Autodesk Inventor part; units mm, degrees
ref_plane "YZ Plane" through (0, 0, 0) normal (1, 0, 0) x (0, 1, 0)
ref_plane "XZ Plane" through (0, 0, 0) normal (0, 1, 0) x (-1, 0, 0)
ref_plane "XY Plane" through (0, 0, 0) normal (0, 0, 1) x (1, 0, 0)
sketch "Sketch1" plane through (0, 0, 0) normal (0, 1, 0) x (-1, 0, 0)
  line L0 (0, 0) -> (-359.4604, 0)
  line L1 (-173.205, -100) -> (23.0868, -100)
  line L2 (23.0868, -100) -> (-382.5472, -100)
  line L3 (-382.5472, -100) -> (-359.4604, 0)
  line L4 (23.0868, -100) -> (0, 0)
  dimension "d16" = 103
  dimension "d17" = 100
  dimension "d18" = 405.634
  dimension "d19" = 103
extrude "Extrusion1" add sketch "Sketch1" along normal blind 5
sketch "Sketch2" plane through (0, 5, 0) normal (0, 1, 0) x (1, 0, 0)
  line L0 (-23.0868, 100) -> (0, 0)
  line L1 (0, 0) -> (-23.0868, 100)
  line L2 (382.5472, 100) -> (-23.0868, 100)
  line L3 (-23.0868, 100) -> (382.5472, 100)
  line L4 (359.4604, 0) -> (382.5472, 100)
  line L5 (382.5472, 100) -> (359.4604, 0)
  line L6 (359.4604, 0) -> (0, 0)
  line L7 (3.9772, 5) -> (-16.801, 95)
  line L8 (-16.801, 95) -> (376.2613, 95)
  line L9 (376.2613, 95) -> (355.4832, 5)
  line L10 (355.4832, 5) -> (3.9772, 5)
  dimension "d6" = 5
extrude "Extrusion2" add sketch "Sketch2" along normal blind 90
sketch "Sketch3" plane through (0, 0, 0) normal (0, 0, 1) x (1, 0, 0)
  line L0 (0, 0) -> (0, 50)
  line L1 (0, 0) -> (0, 95)
  line L2 (0, 50) -> (345.363, 50)
  circle A0 centre (172.6815, 50) radius 7.5
  dimension "d9" = 50
  dimension "d10" = 15
extrude "Extrusion3" cut sketch "Sketch3" against normal blind 455
sketch "Sketch4" plane through (0, 95, 0) normal (0, 1, 0) x (1, 0, 0)
  line L0 (-23.0868, 100) -> (0, 0)
  line L1 (0, 0) -> (-23.0868, 100)
  line L2 (359.4604, 0) -> (382.5472, 100)
  line L3 (-23.0868, 100) -> (382.5472, 100)
  line L4 (382.5472, 100) -> (359.4604, 0)
  line L5 (359.4604, 0) -> (0, 0)
  line L6 (355.4832, 5) -> (3.9772, 5)
extrude "Extrusion4" add sketch "Sketch4" along normal blind 5
properties part number "v chasis" material "Steel, Mild"
Can you work these out from the model? Positions are in its coordinate system, mm. A direction names the side the tool comes from. Give positions to 0.01 mm unless a question says otherwise; leave off trailing zeros. Write each loop counter-clockwise with the first axis right and the second up, starting at its lowest first coordinate (ties: lowest second). Pieces come first, ordered by that corner, then holes. Notation, with made-up numbers: (-8.75, 51) -> (11.25, 51) arc R19 cw to (11.25, 75) -> close; hole circle Ø1 at (-21.75, 80). An arc over 180 degrees is marked (long way). One line per item, written item: value.
Q1. We'd pull the mould along X, two halves only. Please class faces 1 (the face through (370.842, 49.3, -49.3)), 2 (the face through (183, 0, -49)), 3 (the face through (366.018, 49.37, -50.63)): +X half, -X half, draft (parallel to the pull), parting line (faces both ways), or undercut.
Results found:
face 1: +X half
face 2: draft
face 3: undercut
Q2. Imagine slicing it at A-A on y = 50. Please give me the cut outline in (x, z).
Results found:
outline: (-23.09, -100) -> (165.18, -100) -> (165.18, -95) -> (-16.8, -95) -> (3.98, -5) -> (165.18, -5) -> (165.18, 0) -> (0, 0) -> close; (180.18, -100) -> (382.55, -100) -> (359.46, 0) -> (180.18, 0) -> (180.18, -5) -> (355.48, -5) -> (376.26, -95) -> (180.18, -95) -> close
Q3. For P1, Ø1.5, axis at y = 58.5, z = -40, coming from the +X side; P2, Ø4, axis at y = 22, z = -77, coming from the -X side; P3, Ø4, axis at y = 64.5, z = -38, coming from the +X side, each with a flat end and sliding along its axis, tell me the tip position at first contact or that it passes through.
Results found:
P1: stops at x = 368.87
P2: stops at x = -18.24
P3: stops at x = 368.7
Q4. Which directions (+Z, -Z, +X, -X, +Y, -Y) give clear straight access to the entire face, cutting with the end or side of a thin tool? Please do faces 4 (the face through (-6.266, 49.37, -49.37)), 5 (the face through (177, 38, -100)).
Results found:
face 4: none
face 5: -Z, +X, -X, +Y, -Y
Q5. Please list where these lines run through material, in increasing order: line 1 (Z direction, x = 326.5, y = 81); line 2 (Y direction, x = 304.5, z = -15); line 3 (X direction, y = 50, z = -2.75). Write a range as [from, to].
Results found:
line 1: z = [-100, -95], [-5, 0]
line 2: y = [0, 5], [95, 100]
line 3: x = [-0.63, 165.18], [180.18, 360.1]
Q6. Imagine slicing it at C-C on y = 14. Please give me the cut outline in (x, z).
Results found:
outline: (-23.09, -100) -> (382.55, -100) -> (359.46, 0) -> (0, 0) -> close; hole (-16.8, -95) -> (376.26, -95) -> (355.48, -5) -> (3.98, -5) -> close
Q7. Imagine slicing it at B-B on x = 310.5. Please give me the cut outline in (y, z), and give its area (3 significant figures).
Results found:
outline: (0, -100) -> (100, -100) -> (100, 0) -> (0, 0) -> close; hole (5, -95) -> (95, -95) -> (95, -5) -> (5, -5) -> close
area: 1,900 mm^2
